CAD build for the part. Positions are in the model's coordinates, mm. Face numbers are marked on the shaded views. A direction names the side the tool comes from. Round coordinates to 2 decimals unless told otherwise and drop trailing zeros. Write each loop counter-clockwise with the first axis right and the second up, starting at its lowest first coordinate (ties: lowest second). Pieces come first, ordered by that corner, then holes. Notation, with made-up numbers: (37.25, 15) - (82.25, 15) arc R19 ccw to (82.25, 19) - close; hole circle Ø8 at (14.25, 13.25). An arc over 180 degrees is marked (long way). Answer in a Markdown table with one row per item.
```python
from build123d import *

# Parameters (mm, degrees)
F0_W           = 13.375
F0_H           = 2
F1_DEPTH       = 25
F2_R           = 1.75
F3_DEPTH       = 2
F4_W           = 11.3
F4_H           = 13
F5_DEPTH       = 25
F5_DEPTH_BACK  = 11.5
F6_W           = 26
F6_H           = 6.5
F7_DEPTH       = 13
F9_DEPTH       = 13
F11_DEPTH      = 19.75
F11_DEPTH_BACK = 6.25
F13_T1_DEPTH   = 27.75
F13_T3_DEPTH   = 27.75
F13_T5_DEPTH   = 59
F15_DEPTH      = 15
F16_W          = 5.5
F16_H          = 4.8968277758
F16_H_2        = 5.3132384717
F17_DEPTH      = 2
F18_DEPTH      = 2
F19_D          = 3


# Not quite as in the source:
# - a fillet or chamfer that OpenCascade refuses, or shapes differently, is made with other operations: its cross-section is extruded or revolved along the edge and cut away or added


with BuildPart() as f1:
    # F0 (on Right) → F1 (new body, symmetric)
    with BuildSketch(Plane.YZ):
        with Locations((6.6875, 1)):
            Rectangle(F0_W, F0_H)
    extrude(amount=F1_DEPTH, both=True)

    # F2 (on face) → F3 (cut, through all)
    with BuildSketch(Plane.XY.offset(2)):
        with Locations((-13, 4)):
            Circle(F2_R)
        with Locations((13, 4)):
            Circle(F2_R)
    extrude(amount=-F3_DEPTH, mode=Mode.SUBTRACT)

    # F4 (on Right) → F5 (join, two sides)
    with BuildSketch(Plane.YZ) as f5_sk:
        with Locations((-5.65, -4.5)):
            Rectangle(F4_W, F4_H)
    extrude(amount=F5_DEPTH)
    extrude(f5_sk.sketch, amount=-F5_DEPTH_BACK)

    # F6 (on face) → F7 (cut, through all)
    with BuildSketch(Plane(origin=(0, 0, -11), x_dir=(1, 0, 0), z_dir=(0, 0, -1))):
        with Locations((6.75, 8.05)):
            Rectangle(F6_W, F6_H)
    extrude(amount=-F7_DEPTH, mode=Mode.SUBTRACT)

    # F8 (on face) → F9 (cut, through all)
    with BuildSketch(Plane(origin=(0, 0, -11), x_dir=(1, 0, 0), z_dir=(0, 0, -1))):
        Polygon((13, 4.8), (0.5, 4.8), (2.5, 2.8), (11, 2.8), align=None)
    extrude(amount=-F9_DEPTH, mode=Mode.SUBTRACT)

    # F10 (on Right) → F11 (cut, two sides)
    with BuildSketch(Plane.YZ) as f11_sk:
        Polygon((-4.8, -11), (-2.8, -11), (-4.8, 1), align=None)
    extrude(amount=F11_DEPTH, mode=Mode.SUBTRACT)
    extrude(f11_sk.sketch, amount=-F11_DEPTH_BACK, mode=Mode.SUBTRACT)

    # F13: fillet of radius 4.5 on 3 edges, made by hand

    # F13_s2 → F13_t1 (cut)
    with BuildSketch(Plane.YZ.offset(-22.75)):
        with BuildLine():
            ThreePointArc((-6.8, -11), (-9.9819805153, -9.6819805153), (-11.3, -6.5))
            Line((-11.3, -6.5), (-11.3, -11))
            Line((-11.3, -11), (-6.8, -11))
        make_face()
    extrude(amount=F13_T1_DEPTH, mode=Mode.SUBTRACT)

    # F13_s4 → F13_t3 (cut)
    with BuildSketch(Plane.YZ.offset(8.5)):
        with BuildLine():
            ThreePointArc((-6.8, -11), (-9.9819805153, -9.6819805153), (-11.3, -6.5))
            Line((-11.3, -6.5), (-11.3, -11))
            Line((-11.3, -11), (-6.8, -11))
        make_face()
    extrude(amount=F13_T3_DEPTH, mode=Mode.SUBTRACT)

    # F13_s6 → F13_t5 (cut)
    with BuildSketch(Plane.YZ.offset(-22.75)):
        with BuildLine():
            ThreePointArc((0, -6.5), (-1.3180194847, -9.6819805153), (-4.5, -11))
            Line((-4.5, -11), (0, -11))
            Line((0, -11), (0, -6.5))
        make_face()
    extrude(amount=F13_T5_DEPTH, mode=Mode.SUBTRACT)

    # F14 (on face) → F15 (join)
    with BuildSketch(Plane.XY.offset(2)):
        Polygon((25, 0), (-11.5, 0), (-11.5, -11.3), (-6.25, -11.3), (-6.25, -4.8), (0.5, -4.8), (2.5, -2.8), (11, -2.8), (13, -4.8), (19.75, -4.8), (19.75, -11.3), (25, -11.3), align=None)
    extrude(amount=F15_DEPTH)

    # F16 (on face) → F17 (join)
    with BuildSketch(Plane(origin=(0, 0, 0), x_dir=(-1, 0, 0), z_dir=(0, 1, 0))):
        with Locations((-16.04918, 4.4484138879)):
            Rectangle(F16_W, F16_H)
        with Locations((2.45082, 4.6566192359)):
            Rectangle(F16_W, F16_H_2)
    extrude(amount=-F17_DEPTH)

    # F16 (on face) → F18 (cut)
    with BuildSketch(Plane(origin=(0, 0, 0), x_dir=(-1, 0, 0), z_dir=(0, 1, 0))):
        with Locations((-16.04918, 4.4484138879)):
            Rectangle(F16_W, F16_H)
        with Locations((2.45082, 4.6566192359)):
            Rectangle(F16_W, F16_H_2)
    extrude(amount=-F18_DEPTH, mode=Mode.SUBTRACT)

    # F19 (through all)
    with Locations(Plane.XZ.offset(4.8)):
        with Locations((16, 4), (-2.5, 4)):
            Hole(F19_D / 2)


solid = f1.part
```
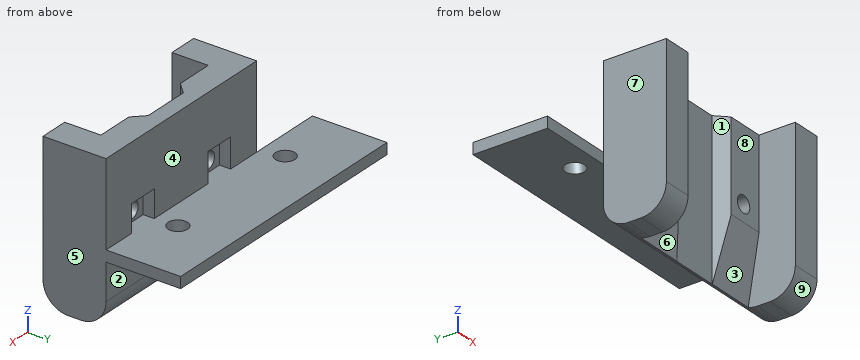
Q1. Flat gauge pins, fed straight in: pin 1 (3.5 mm diameter, centred on y = -7, z = 9, fed in from -X); pin 2 (1.6 mm diameter, centred on x = -20.5, z = 1.5, fed in from -Y); pin 3 (9.5 mm diameter, centred on x = 5, z = 8.5, fed in from -Y); pin 4 (7 mm diameter, centred on x = 6.5, z = -3, fed in from +Y) (3 decimals). Where does each tip first touch, or does it go through?
Computed:
| item | result |
|---|---|
| pin 1 | stops at x = -11.5 |
| pin 2 | stops at y = 0 |
| pin 3 | stops at y = -4.8 |
| pin 4 | stops at y = 13.375 |
Q2. Pull direction X, two halves, no side cores. Call the marked faces 6, 7, 8 and 9: released by +X, released by -X, zero draft, split by the parting line, or undercut.
Computed:
| item | result |
|---|---|
| face 6 | undercut |
| face 7 | released by -X |
| face 8 | undercut |
| face 9 | zero draft |
Q3. Saw through at A-A on x = -2.5. List the corners of the cut face in (y, z) (3 decimals).
Computed:
| item | result |
|---|---|
| outline | (-4.8, 1) - (-2.852, -10.687) arc R4.5 ccw to (0, -6.5) - (0, 0) - (13.375, 0) - (13.375, 2) - (-2, 2) - (-2, 2.5) - (-4.8, 2.5) - close; (-4.8, 5.5) - (-2, 5.5) - (-2, 7.313) - (0, 7.313) - (0, 17) - (-4.8, 17) - close |
Q4. Saw through at B-B on z = 4. List the corners of the cut face in (x, y).
Computed:
| item | result |
|---|---|
| outline | (-11.5, -11.3) - (-6.25, -11.3) - (-6.25, -4.8) - (-4, -4.8) - (-4, -2) - (-5.2, -2) - (-5.2, 0) - (-11.5, 0) - close; (-1, -4.8) - (0.5, -4.8) - (2.5, -2.8) - (11, -2.8) - (13, -4.8) - (14.5, -4.8) - (14.5, -2) - (13.3, -2) - (13.3, 0) - (0.3, 0) - (0.3, -2) - (-1, -2) - close; (17.5, -4.8) - (19.75, -4.8) - (19.75, -11.3) - (25, -11.3) - (25, 0) - (18.8, 0) - (18.8, -2) - (17.5, -2) - close |
Q5. Drill centre lines: line 1 (X direction, y = -1.5, z = 5.25); line 2 (X direction, y = -9.75, z = -7); line 3 (Y direction, x = -13, z = 0.8) (3 decimals). Where is each one in solid material? Low to high.
Computed:
| item | result |
|---|---|
| line 1 | x = -11.5 to -5.2, 0.3 to 13.3, 18.8 to 25 |
| line 2 | x = -11.5 to -6.25, 19.75 to 25 |
| line 3 | y = 0 to 2.25, 5.75 to 13.375 |
Q6. Saw through at D-D on y = -5.75. List the corners of the cut face in (x, z), then the cut area to 3 significant figures.
Computed:
| item | result |
|---|---|
| outline | (-11.5, -11) - (-6.25, -11) - (-6.25, 17) - (-11.5, 17) - close; (19.75, -11) - (25, -11) - (25, 17) - (19.75, 17) - close |
| area | 294 mm2 |
Q7. 3-axis set-ups, long thin cutter, end or side, ignore diameter. For the marked faces 1, 2, 3, 4 and 5: which of +Z, -Z, +X, -X, +Y, -Y reach the whole face in a straight line?
Computed:
| item | result |
|---|---|
| face 1 | +Z, -Z, -Y |
| face 2 | -Z, +X, -X, +Y |
| face 3 | -Z, -Y |
| face 4 | +Z, +X, -X, +Y |
| face 5 | +Z, -Z, +X, +Y, -Y |
Q8. Saw through at C-C on y = 4. List the corners of the cut face in (x, z).
Computed:
| item | result |
|---|---|
| outline | (-25, 0) - (-14.75, 0) - (-14.75, 2) - (-25, 2) - close; (-11.25, 0) - (11.25, 0) - (11.25, 2) - (-11.25, 2) - close; (14.75, 0) - (25, 0) - (25, 2) - (14.75, 2) - close |
